Autodesk Inventor part; units mm, degrees
ref_plane "YZ Plane" through (0, 0, 0) normal (1, 0, 0) x (0, 1, 0)
ref_plane "XZ Plane" through (0, 0, 0) normal (0, 1, 0) x (-1, 0, 0)
ref_plane "XY Plane" through (0, 0, 0) normal (0, 0, 1) x (1, 0, 0)
sketch "Sketch1" plane through (0, 0, 0) normal (0, 0, 1) x (1, 0, 0)
  circle A0 centre (0, 0) radius 24.75
  circle A1 centre (0, 0) radius 12.5
  dimension "d0" = 49.5
  dimension "d1" = 25
extrude "Extrusion1" add sketch "Sketch1" along normal blind 22
sketch "Sketch3" plane through (0, 0, 0) normal (0, 0, -1) x (-1, 0, 0)
  circle A0 centre (0, 0) radius 24.75
  circle A1 centre (0, 0) radius 27.5
  dimension "d13" = 49.5
  dimension "d14" = 55
extrude "Extrusion3" add sketch "Sketch3" against normal blind 5
sketch "Sketch2" plane through (0, 0, 22) normal (0, 0, 1) x (1, 0, 0)
  circle A0 centre (15, 0) radius 11
  point P0 (0, 0)
  dimension "d4" = 15
  dimension "d5" = 0
  dimension "d6" = 22
extrude "Extrusion2" cut sketch "Sketch2" against normal blind 22
fillet "Fillet1" radius 2 4 edges at (8.675, 8.9997, 11) (8.675, -8.9997, 11) (23.8854, -6.4845, 13.5) (23.8854, 6.4845, 13.5)
pattern_circular "Circular Pattern1" count 3 over 360 about axis through (0, 0, 0) along (0, 0, 1) of "Extrusion2", "Fillet1"
sketch "Sketch4" plane through (0, 0, 22) normal (0, 0, 1) x (1, 0, 0)
  circle A0 centre (9, -16) radius 1.75
  point P0 (0, 0)
  dimension "d17" = 3.5
  dimension "d18" = 16
  dimension "d19" = 9
extrude "Extrusion4" cut sketch "Sketch4" against normal through all
pattern_circular "Circular Pattern2" count 3 over 360 about axis through (0, 0, 0) along (0, 0, 1) of "Extrusion4"
properties part number "LayerBase2"
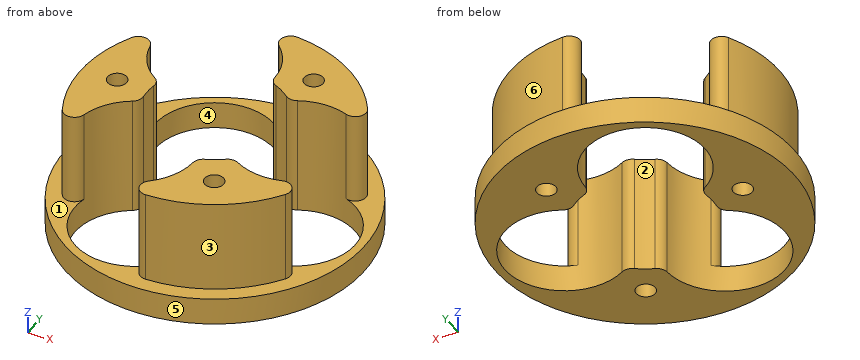
Verification items for the finished model (mm, model axes). Face numbers are marked on the shaded views. A direction names the side the tool comes from. Give positions to 0.01 mm unless a question says otherwise; leave off trailing zeros. Write each loop counter-clockwise with the first axis right and the second up, starting at its lowest first coordinate (ties: lowest second). Pieces come first, ordered by that corner, then holes.
(1) Cross-section at C-C (z = 8.25). State how many separate pieces and enclosed holes the cut face has, plus the area to 3 significant figures.
(2) Cross-section at B-B (x = 15). Enter the section's corners in (y, z), plus the area to 3 significant figures.
(3) Gauge pin test, flat ends, axial feed: pin 1 (20 mm diameter, centred on x = -7.5, y = 12.99, fed in from -Z); pin 2 (4 mm diameter, centred on y = -11, z = 11.5, fed in from +X); pin 3 (12 mm diameter, centred on x = -6.5, z = 17, fed in from -Y); pin 4 (12 mm diameter, centred on x = 19.5, z = 12, fed in from -Y). Record the tip position at first contact, or that the pin passes through.
(4) Cross-section at D-D (x = -15). Enter the section's corners in (y, z), plus the area to 3 significant figures.
(5) Mould release check, pull along X, two halves, no side actions. Record for the marked faces 4, 5 and 6: +X half, -X half, draft (parallel to the pull), parting line (faces both ways), or undercut.
(6) Access from +Z, -Z, +X, -X, +Y, -Y to the whole of each face (thin tool, end or side, straight path). Record for the marked faces 1, 2 and 3.
(7) Material ranges on line 1 (X direction, y = 14.5, z = 1.5); line 2 (Z direction, x = 20, y = 17.5); line 3 (Y direction, x = 15, z = 6.75), recorded low to high.
(8) Cross-section at A-A (y = 15). Enter the section's corners in (x, z).
Worked out:
1. separate pieces: 3
1. enclosed holes: 3
1. area: 567 mm2
2. outline: (-23.05, 0) - (-11, 0) - (-11, 22) - (-19.69, 22) - (-19.69, 5) - (-23.05, 5) - close; (11, 0) - (23.05, 0) - (23.05, 5) - (19.69, 5) - (19.69, 22) - (11, 22) - close
2. area: 416 mm2
3. pin 1: passes through
3. pin 2: stops at x = 21.12
3. pin 3: stops at y = -23.9
3. pin 4: stops at y = -20.74
4. outline: (-23.05, 0) - (-21.04, 0) - (-21.04, 5) - (-23.05, 5) - close; (-4.94, 0) - (4.94, 0) - (4.94, 22) - (-4.94, 22) - close; (21.04, 0) - (23.05, 0) - (23.05, 5) - (21.04, 5) - close
4. area: 238 mm2
5. face 4: undercut
5. face 5: parting line
5. face 6: +X half
6. face 1: +Z
6. face 2: +Z, -Z
6. face 3: +Z, +X, -Y
7. line 1: x = -23.37 to -18.4, 3.4 to 8.18, 10.53 to 23.37
7. line 2: z = 0 to 5
7. line 3: y = -19.69 to -11, 11 to 19.69
8. outline: (-23.05, 0) - (-18.31, 0) - (-18.31, 5) - (-23.05, 5) - close; (3.31, 0) - (7.8, 0) - (7.8, 22) - (3.31, 22) - close; (10.92, 0) - (23.05, 0) - (23.05, 5) - (19.69, 5) - (19.69, 22) - (10.92, 22) - close
